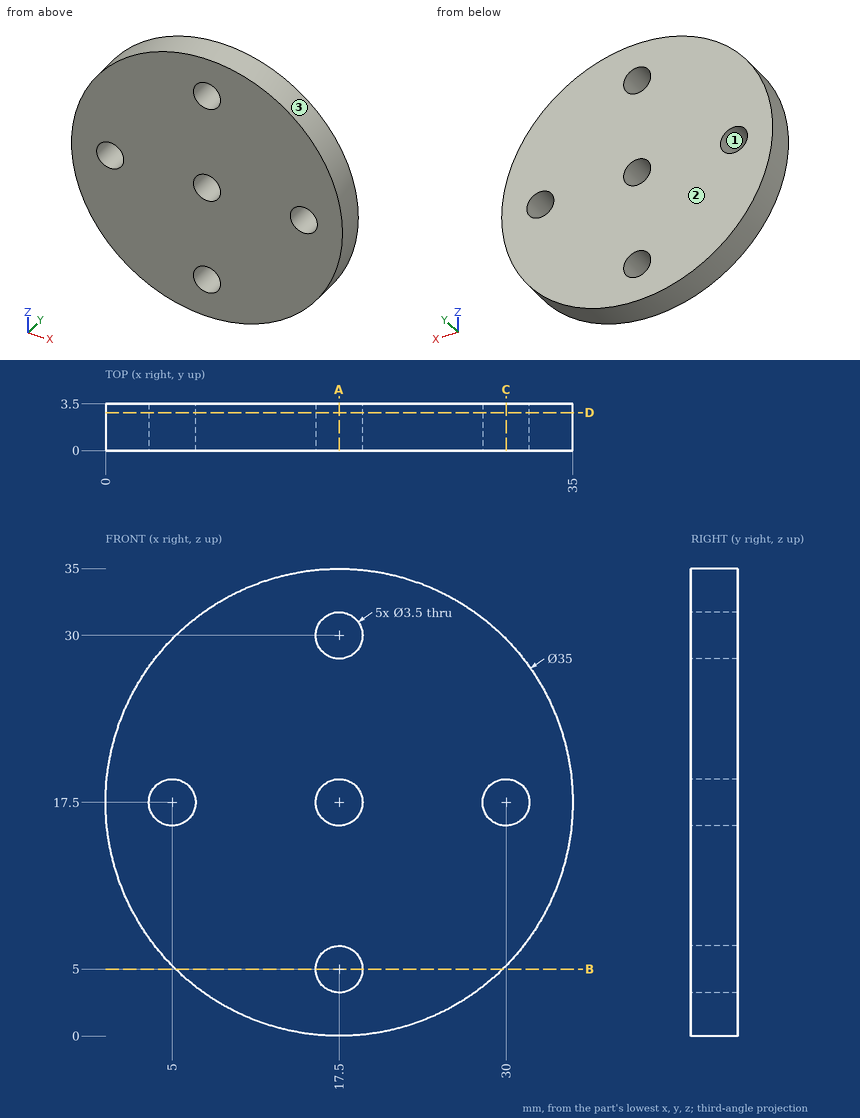
Can you work these out from the drawing? Everything is in mm from the part's minimum corner. Round coordinates to 2 decimals unless told otherwise and drop trailing zeros. Loops run counter-clockwise (first coordinate to the right, second up) from the corner with the lowest first, then second, coordinate; pieces in that order, holes last. Notation, with made-up numbers: (-19.5, 29) -> (15.5, 29) arc R19 cw to (15.5, 39) -> close; hole circle Ø4 at (48.25, -20.5). An arc over 180 degrees is marked (long way). Use CSV: the item, a comma, the result in double quotes.
(1) Suppose I cut it at D-D on y = 2.85. Write out the boundary of the cut face in (x, z).
Return value:
outline,"circle Ø35 at (17.5, 17.5); hole circle Ø3.5 at (5, 17.5); hole circle Ø3.5 at (17.5, 5); hole circle Ø3.5 at (17.5, 17.5); hole circle Ø3.5 at (17.5, 30); hole circle Ø3.5 at (30, 17.5)"
(2) Will this pin go through, and if not, where does the flat tip stop? pin 1 Ø4.5 at (x, z) = (17.5, 17.5) entering from +Y.
Return value:
pin 1,"stops at y = 3.5"
(3) If I drill on probe 1 along X at (y, z) = (1, 17.5); probe 2 along X at (y, z) = (0.2, 19), over which ranges is the centre line in solid material (lowest first)? Write a range as [from, to].
Return value:
probe 1,"x = [0, 3.25], [6.75, 15.75], [19.25, 28.25], [31.75, 35]"
probe 2,"x = [0.06, 4.1], [5.9, 16.6], [18.4, 29.1], [30.9, 34.94]"
(4) Suppose I cut it at C-C on x = 30. Write out the boundary of the cut face in (y, z).
Return value:
outline,"(0, 5.25) -> (3.5, 5.25) -> (3.5, 15.75) -> (0, 15.75) -> close; (0, 19.25) -> (3.5, 19.25) -> (3.5, 29.75) -> (0, 29.75) -> close"
(5) Suppose I cut it at B-B on z = 5. Write out the boundary of the cut face in (x, y).
Return value:
outline,"(5.25, 0) -> (15.75, 0) -> (15.75, 3.5) -> (5.25, 3.5) -> close; (19.25, 0) -> (29.75, 0) -> (29.75, 3.5) -> (19.25, 3.5) -> close"
(6) Suppose I cut it at A-A on x = 17.5. Write out the boundary of the cut face in (y, z).
Return value:
outline,"(0, 0) -> (3.5, 0) -> (3.5, 3.25) -> (0, 3.25) -> close; (0, 6.75) -> (3.5, 6.75) -> (3.5, 15.75) -> (0, 15.75) -> close; (0, 19.25) -> (3.5, 19.25) -> (3.5, 28.25) -> (0, 28.25) -> close; (0, 31.75) -> (3.5, 31.75) -> (3.5, 35) -> (0, 35) -> close"
(7) If we mould it in two halves opening along Z, with no side actions, what happens to the marked faces 1, 2 and 3? For each: +Z half, -Z half, draft (parallel to the pull), parting line (faces both ways), or undercut.
Return value:
face 1,"undercut"
face 2,"draft"
face 3,"parting line"
